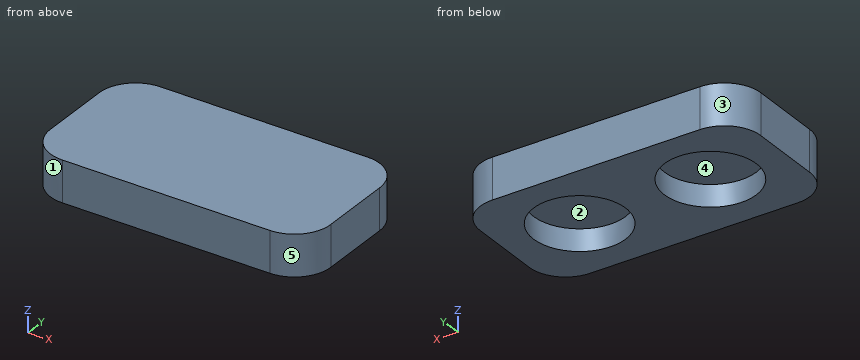
```python
from build123d import *

# Parameters (mm, degrees)
F0_R     = 1.9
F1_DEPTH = 1.7
F2_R     = 1.9
F3_DEPTH = 0.8


# Not quite as in the source:
# - a feature names something its author has since deleted; it is built from what else it names


with BuildPart() as f1:
    # F0 (on Top) → F1 (new body)
    with BuildSketch(Plane.XY):
        with BuildLine():
            Line((-0.3902956496, 3), (-4.2902956496, 3))
            ThreePointArc((-4.2902956496, 3), (-5.3509558214, 2.5606601718), (-5.7902956496, 1.5))
            Line((-5.7902956496, 1.5), (-5.7902956496, -1.5))
            ThreePointArc((-5.7902956496, -1.5), (-5.3509558214, -2.5606601718), (-4.2902956496, -3))
            Line((-4.2902956496, -3), (-0.3902956496, -3))
            Line((-0.3902956496, -3), (0.3902956496, -3))
            Line((0.3902956496, -3), (4.2902956496, -3))
            ThreePointArc((4.2902956496, -3), (5.3509558214, -2.5606601718), (5.7902956496, -1.5))
            Line((5.7902956496, -1.5), (5.7902956496, 1.5))
            ThreePointArc((5.7902956496, 1.5), (5.3509558214, 2.5606601718), (4.2902956496, 3))
            Line((4.2902956496, 3), (0.3902956496, 3))
            Line((0.3902956496, 3), (-0.3902956496, 3))
        make_face()
        with Locations((-2.7, 0)):
            Circle(F0_R, mode=Mode.SUBTRACT)
        with Locations((2.7, 0)):
            Circle(F0_R, mode=Mode.SUBTRACT)
    extrude(amount=F1_DEPTH)

    # F2 (on face) → F3 (join)
    with BuildSketch(Plane.XY.offset(1.7)):
        with BuildLine():
            ThreePointArc((-5.7902956496, -1.5), (-5.3509558214, -2.5606601718), (-4.2902956496, -3))
            Line((-4.2902956496, -3), (4.2902956496, -3))
            ThreePointArc((4.2902956496, -3), (5.3509558214, -2.5606601718), (5.7902956496, -1.5))
            Line((5.7902956496, -1.5), (5.7902956496, 1.5))
            ThreePointArc((5.7902956496, 1.5), (5.3509558214, 2.5606601718), (4.2902956496, 3))
            Line((4.2902956496, 3), (-4.2902956496, 3))
            ThreePointArc((-4.2902956496, 3), (-5.3509558214, 2.5606601718), (-5.7902956496, 1.5))
            Line((-5.7902956496, 1.5), (-5.7902956496, -1.5))
        make_face()
        with Locations((-2.7, 0)):
            Circle(F2_R, mode=Mode.SUBTRACT)
        with Locations((2.7, 0)):
            Circle(F2_R, mode=Mode.SUBTRACT)
        with Locations((-2.7, 0)):
            Circle(F2_R)
        with Locations((2.7, 0)):
            Circle(F2_R)
    extrude(amount=-F3_DEPTH)


solid = f1.part
```
Work out the finished part from the listing and answer in its coordinate system (mm). Face numbers are marked on the shaded views. A direction names the side the tool comes from. Round coordinates to 2 decimals unless told otherwise and drop trailing zeros. Write each loop counter-clockwise with the first axis right and the second up, starting at its lowest first coordinate (ties: lowest second). Pieces come first, ordered by that corner, then holes. Notation, with made-up numbers: (75.25, 45) - (133.25, 45) arc R13 ccw to (133.25, 51) - close; hole circle Ø5 at (-0.75, 87). An arc over 180 degrees is marked (long way). Return JSON: item names as keys, results as strings. Group by question number.
Q1. The part is cut by section A-A on z = 0.75. Write down the section's boundary in (x, y), then the cut area to 3 significant figures.
Q2. Find the intervals of material crossed by L1, parallel to X at y = 0, z = 0.4; L2, parallel to X at y = -0.9, z = 0.4; L3, parallel to Y at x = -2.7, z = 0.6, in increasing order.
Q3. The mould has two halves that part along X. Classify the marked faces 3, 4 and 5: released by +X, released by -X, zero draft, split by the parting line, or undercut.
Q4. This flat-tipped pin is pushed along its axis until it touches: pin 1 Ø1.1 at (x, y) = (-3, -0.5) entering from -Z. Where does it stop, or does it pass through?
Q5. The part is cut by section B-B on x = -2.7. Write down the section's boundary in (y, z), then the cut area to 3 significant figures.
Q6. For the marked faces 1 and 2, determine the directions among +Z, -Z, +X, -X, +Y, -Y from which every point of the face is accessible in a straight line to the end or side of a thin tool.
Q7. The part is cut by section D-D on y = 1.65. Write down the section's boundary in (x, z).
Q8. The part is cut by section C-C on y = 0. Write down the section's boundary in (x, z).
Solved:
{
 "1": {"outline": "(-5.79, -1.5) arc R1.5 ccw to (-4.29, -3) - (4.29, -3) arc R1.5 ccw to (5.79, -1.5) - (5.79, 1.5) arc R1.5 ccw to (4.29, 3) - (-4.29, 3) arc R1.5 ccw to (-5.79, 1.5) - close; hole circle Ø3.8 at (-2.7, 0); hole circle Ø3.8 at (2.7, 0)", "area": "44.9 mm²"},
 "2": {"L1": "-5.79 to -4.6, -0.8 to 0.8, 4.6 to 5.79", "L2": "-5.79 to -4.37, -1.03 to 1.03, 4.37 to 5.79", "L3": "-3 to -1.9, 1.9 to 3"},
 "3": {"face 3": "released by -X", "face 4": "undercut", "face 5": "released by +X"},
 "4": {"pin 1": "z = 0.9"},
 "5": {"outline": "(-3, 0) - (-1.9, 0) - (-1.9, 0.9) - (1.9, 0.9) - (1.9, 0) - (3, 0) - (3, 1.7) - (-3, 1.7) - close", "area": "6.78 mm²"},
 "6": {"face 1": "+Z, -Z, -X, -Y", "face 2": "-Z"},
 "7": {"outline": "(-5.78, 0) - (-3.64, 0) - (-3.64, 0.9) - (-1.76, 0.9) - (-1.76, 0) - (1.76, 0) - (1.76, 0.9) - (3.64, 0.9) - (3.64, 0) - (5.78, 0) - (5.78, 1.7) - (-5.78, 1.7) - close"},
 "8": {"outline": "(-5.79, 0) - (-4.6, 0) - (-4.6, 0.9) - (-0.8, 0.9) - (-0.8, 0) - (0.8, 0) - (0.8, 0.9) - (4.6, 0.9) - (4.6, 0) - (5.79, 0) - (5.79, 1.7) - (-5.79, 1.7) - close"}
}
